Build history of the part. All positions in model axes, mm. A direction names the side the tool comes from. Coordinates: 2 decimals unless noted, no trailing zeros. Order: outer loops, then holes, each group sorted by start corner. A loop starts at its lowest first (then second) coordinate and runs counter-clockwise, first axis right, second up. Notation, with made-up numbers: (44.5, 6) - (80.5, 6) arc R8 ccw to (80.5, 19) - close; hole circle Ø11 at (-7.5, -38). An arc over 180 degrees is marked (long way). One line per item, written item: value.
from build123d import *

# Parameters (mm, degrees)
CYLINDER001_R     = 0.44
CYLINDER001_DEPTH = 3
CYLINDER_R        = 0.44
CYLINDER_DEPTH    = 3
BOX_W             = 17.5
BOX_H             = 7
BOX_DEPTH         = 13.5
FILLET_R          = 0.5


with BuildPart() as pin2:
    # Cylinder001 → Cylinder001 (new body)
    with BuildSketch(Plane(origin=(7.5, 0, -3), x_dir=(1, 0, 0), z_dir=(0, 0, 1))):
        Circle(CYLINDER001_R)
    extrude(amount=CYLINDER001_DEPTH)


with BuildPart() as pin1:
    # Cylinder → Cylinder (new body)
    with BuildSketch(Plane(origin=(-7.5, 0, -3), x_dir=(1, 0, 0), z_dir=(0, 0, 1))):
        Circle(CYLINDER_R)
    extrude(amount=CYLINDER_DEPTH)


with BuildPart() as obj1:
    # Box → Box (new body)
    with BuildSketch(Plane(origin=(-8.75, -3.5, 0), x_dir=(1, 0, 0), z_dir=(0, 0, 1))):
        with Locations((8.75, 3.5)):
            Rectangle(BOX_W, BOX_H)
    extrude(amount=BOX_DEPTH)

    # Fillet
    fillet_edges = [obj1.edges().sort_by_distance(p)[0] for p in [
        (-8.75, -3.5, 6.75),
        (-8.75, 0, 13.5),
        (-8.75, 3.5, 6.75),
        (8.75, -3.5, 6.75),
        (8.75, 0, 13.5),
        (8.75, 3.5, 6.75),
        (0, -3.5, 13.5),
        (0, 3.5, 13.5),
    ]]
    fillet(fillet_edges, radius=FILLET_R)

    # Fusion: union Pin1
    add(pin1.part)

    # Fusion001: union Pin2
    add(pin2.part)


solid = obj1.part
1. Two-plate mould, pull along X, no slides. Class faces 3 (the face through (-8.75, 0, 6)), 4 (the face through (0, 3.5, 6)), 5 (the face through (-7.094, -0.169, -1.521)): pulls with the +X half, pulls with the -X half, needs draft (parallel to the pull), parting line crosses it, or undercut.
Values found:
face 3: pulls with the -X half
face 4: needs draft
face 5: undercut
2. Band-saw the part on A-A, the plane y = -1. Give the cut face in (x, z).
Values found:
outline: (-8.75, 0) - (8.75, 0) - (8.75, 13) arc R0.5 ccw to (8.25, 13.5) - (-8.25, 13.5) arc R0.5 ccw to (-8.75, 13) - close
3. Probe line 1 along Z through (x, y) = (-6.25, 0.75); line 2 along Z through (x, y) = (1.75, 3.25). List the from-to ranges inside material, lowest first.
Values found:
line 1: z = 0 to 13.5
line 2: z = 0 to 13.43
4. Band-saw the part on C-C, the plane x = 2. Give the cut face in (y, z), and give its area (3 significant figures).
Values found:
outline: (-3.5, 0) - (3.5, 0) - (3.5, 13) arc R0.5 ccw to (3, 13.5) - (-3, 13.5) arc R0.5 ccw to (-3.5, 13) - close
area: 94.4 mm2
5. Band-saw the part on B-B, the plane x = -7.5. Give the cut face in (y, z).
Values found:
outline: (-3.5, 0) - (-0.44, 0) - (-0.44, -3) - (0.44, -3) - (0.44, 0) - (3.5, 0) - (3.5, 13) arc R0.5 ccw to (3, 13.5) - (-3, 13.5) arc R0.5 ccw to (-3.5, 13) - close
6. Flat gauge pin, fed straight in: P1, Ø2, axis at x = -3.5, y = 1, coming from the -Z side. Where does the tip first touch, or does it go through?
Values found:
P1: stops at z = 0
7. Band-saw the part on D-D, the plane y = 0. Give the cut face in (x, z), and give its area (3 significant figures).
Values found:
outline: (-8.75, 0) - (-7.94, 0) - (-7.94, -3) - (-7.06, -3) - (-7.06, 0) - (7.06, 0) - (7.06, -3) - (7.94, -3) - (7.94, 0) - (8.75, 0) - (8.75, 13) arc R0.5 ccw to (8.25, 13.5) - (-8.25, 13.5) arc R0.5 ccw to (-8.75, 13) - close
area: 241 mm2
8. 3-axis set-ups, long thin cutter, end or side, ignore diameter. For faces 1 (the face through (-7.5, 0, -3)), 2 (the face through (7.906, -0.169, -1.521)): which of +Z, -Z, +X, -X, +Y, -Y reach the whole face in a straight line?
Values found:
face 1: -Z, +X, -X, +Y, -Y
face 2: -Z
